The listing builds one solid part. Answer for the finished solid, in the listing's coordinates (mm). A direction names the side the tool comes from. Give positions to 0.01 mm unless a question says otherwise; leave off trailing zeros. Write each loop counter-clockwise with the first axis right and the second up, starting at its lowest first coordinate (ties: lowest second). Pieces come first, ordered by that corner, then holes. Notation, with made-up numbers: (0, 28.5) - (10, 28.5) arc R23 ccw to (10, 63.5) - close; hole circle Ø2 at (49.5, 46.5). An arc over 180 degrees is marked (long way). One line per item, written item: value. Start each with the question number.
Autodesk Inventor part; units mm, degrees
ref_plane "YZ Plane" through (0, 0, 0) normal (1, 0, 0) x (0, 1, 0)
ref_plane "XZ Plane" through (0, 0, 0) normal (0, 1, 0) x (-1, 0, 0)
ref_plane "XY Plane" through (0, 0, 0) normal (0, 0, 1) x (1, 0, 0)
sketch "Sketch1" plane through (0, 0, 0) normal (0, 0, 1) x (1, 0, 0)
  line L0 (0, 0) -> (230, 0)
  line L1 (230, 0) -> (230, 338.262)
  line L2 (230, 338.262) -> (0, 338.262)
  line L3 (0, 338.262) -> (0, 0)
  line L4 (39.012, 39.012) -> (190.988, 39.012)
  line L5 (190.988, 39.012) -> (190.988, 300.162)
  line L6 (190.988, 300.162) -> (39.012, 300.162)
  line L7 (39.012, 300.162) -> (39.012, 39.012)
  dimension "d0" = 230
  dimension "d1" = 338.262
  dimension "d2" = 39.012
  dimension "d3" = 39.012
  dimension "d4" = 39.012
  dimension "d5" = 38.1
extrude "Extrusion1" add sketch "Sketch1" along normal blind 6.35
fillet "Fillet2" radius 25.4 4 edges at (190.988, 39.012, 3.175) (39.012, 39.012, 3.175) (39.012, 300.162, 3.175) (190.988, 300.162, 3.175)
thicken "Thicken1" operation add thickness 3 both sides no extend neighbours yes toward (-1, 0, 0) faces at (39.012, 134.5287, 4.2333) (98.1373, 300.162, 2.1167) (190.988, 204.6453, 4.2333) (131.8627, 39.012, 2.1167) (184.2075, 47.1356, 2.1167) (60.6263, 39.2957, 2.1167) (40.7678, 284.0417, 2.1167) (189.2322, 284.0417, 2.1167)
equation "\"d3\" = d2"
equation "\"d4\" = d2"
properties part number "Door Panel Front Foam" material "Polyurethane Foam"
Item 1: This flat-tipped pin is pushed along its axis until it touches: pin 1 Ø2 at (x, z) = (50.5, 4) entering from -Y. Where does it stop, or does it pass through?
Item 2: Find section B-B on y = 113. Determine the outline of the cut face in (x, z), plus the area to 3 significant figures.
Item 3: Straight lines are drawn through the part: line 1 along X through (y, z) = (68, 2.5); line 2 along Y through (x, z) = (148.5, 6); line 3 along X through (y, z) = (50.5, 5.5). For each, find the intervals that lie inside material, in ascending order.
Item 4: Find section A-A on z = 4.75. Determine the outline of the cut face in (x, y).
Item 5: Find section C-C on x = 126. Determine the outline of the cut face in (y, z), plus the area to 3 significant figures.
Item 6: The mould has two halves that part along X. Classify faces 3 (the flat face through (230, 167, 3)), 4 (the flat face through (116, 303.162, 3)), 5 (the flat face through (117, 338.262, 3)): +X half, -X half, draft (parallel to the pull), parting line (faces both ways), or undercut.
Item 7: For faces 1 (the cylindrical face through (185.45, 44.11, 3.22)), 2 (the flat face through (113, 0, 3)), determine the directions among +Z, -Z, +X, -X, +Y, -Y from which every point of the face is accessible in a straight line to the end or side of a thin tool.
Values:
1. pin 1: y = 0
2. outline: (0, 0) - (36.01, 0) - (36.01, 6.35) - (0, 6.35) - close; (193.99, 0) - (230, 0) - (230, 6.35) - (193.99, 6.35) - close
2. area: 457 mm^2
3. line 1: 0 to 36.01, 193.99 to 230
3. line 2: 0 to 36.01, 303.16 to 338.26
3. line 3: 0 to 39.65, 190.35 to 230
4. outline: (0, 0) - (230, 0) - (230, 338.26) - (0, 338.26) - close; hole (36.01, 64.41) arc R28.4 ccw to (64.41, 36.01) - (165.59, 36.01) arc R28.4 ccw to (193.99, 64.41) - (193.99, 274.76) arc R28.4 ccw to (165.59, 303.16) - (64.41, 303.16) arc R28.4 ccw to (36.01, 274.76) - close
5. outline: (0, 0) - (36.01, 0) - (36.01, 6.35) - (0, 6.35) - close; (303.16, 0) - (338.26, 0) - (338.26, 6.35) - (303.16, 6.35) - close
5. area: 452 mm^2
6. face 3: +X half
6. face 4: undercut
6. face 5: draft
7. face 1: +Z, -Z
7. face 2: +Z, -Z, +X, -X, -Y
